Can you work these out from the model? Positions are in its coordinate system, mm. A direction names the side the tool comes from. Round coordinates to 2 decimals unless told otherwise and drop trailing zeros. Write each loop counter-clockwise with the first axis right and the second up, starting at its lowest first coordinate (ties: lowest second). Pieces come first, ordered by that corner, then holes. Notation, with made-up numbers: (48, 56.5) - (89, 56.5) arc R37 ccw to (89, 92.5) - close; hole circle Ø4 at (-29.75, 72.25). An arc over 180 degrees is marked (long way). One line per item, written item: value. Start each with the question number.
(1) On a 3-axis mill with a long thin cutter (end or side, diameter ignored), from which of +Z, -Z, +X, -X, +Y, -Y can I reach the whole of each face in a straight line? I mean faces 1 (the face through (-33, 0, 77.986)), 2 (the face through (-16.92, -0.07, 51.26)). Say none if no direction works.
(2) I want a section at D-D on z = 35. List the corners of the cut face in (x, y) for me.
(3) If I drill on L1, parallel to X at y = -2.5, z = 9; L2, parallel to X at y = -1, z = 51, over which ranges is the centre line in solid material (lowest first)? Write a range as from..to.
(4) I'm going to push a flat-ended pin straight in: pin 1 Ø2 at (y, z) = (-3.5, 18.5) entering from +X. Where does the tip first touch, or does it pass through?
(5) I want a section at C-C on x = -19. Give the number of separate pieces and of enclosed holes in the cut face, plus the area to 3 significant figures.
(6) Thinking about a two-plate mould opening in Z: for faces 3 (the face through (-30, -5.08, 3)), 4 (the face through (-16.9, -0.1, 20.8)), 5 (the face through (-16.92, -0.07, -24.94)), 6 (the face through (-16.81, -0.07, 74.12)), which applies, +Z half, -Z half, draft (parallel to the pull), parting line (faces both ways), or undercut?
(7) I want a section at B-B on z = 5.5. List the corners of the cut face in (x, y) for me, plus the area to 3 significant figures.
(8) I want a section at A-A on y = 0.25. List the corners of the cut face in (x, z) for me, plus the area to 3 significant figures.
from build123d import *

# Parameters (mm, degrees)
F1_DEPTH = 5.08


with BuildPart() as f1:
    # F0 (on Front) → F1 (new body, symmetric)
    with BuildSketch(Plane.XZ):
        Polygon((-20.673906, 77.98629), (-46.073906, 77.98629), (-46.073906, -74.41371), (-20.673906, -74.41371), (-13.053906, -66.79371), (-20.673906, -59.17371), (-13.053906, -51.55371), (-20.673906, -43.93371), (-13.053906, -36.31371), (-20.673906, -28.69371), (-13.053906, -21.07371), (-20.673906, -13.45371), (-13.053906, -5.83371), (-20.673906, 1.78629), (-13.053906, 9.40629), (-20.673906, 17.02629), (-13.053906, 24.64629), (-20.673906, 32.26629), (-13.053906, 39.88629), (-20.673906, 47.50629), (-13.053906, 55.12629), (-20.673906, 62.74629), (-13.053906, 70.36629), align=None)
    extrude(amount=F1_DEPTH, both=True)


solid = f1.part
Established:
1. face 1: +Z, +X, -X, +Y, -Y
1. face 2: +X, +Y, -Y
2. outline: (-46.07, -5.08) - (-17.94, -5.08) - (-17.94, 5.08) - (-46.07, 5.08) - close
3. L1: -46.07..-13.46
3. L2: -46.07..-17.18
4. pin 1: x = -18.2
5. separate pieces: 10
5. enclosed holes: 0
5. area: 1,210 mm2
6. face 3: draft
6. face 4: undercut
6. face 5: undercut
6. face 6: +Z half
7. outline: (-46.07, -5.08) - (-16.96, -5.08) - (-16.96, 5.08) - (-46.07, 5.08) - close
7. area: 296 mm2
8. outline: (-46.07, -74.41) - (-20.67, -74.41) - (-13.05, -66.79) - (-20.67, -59.17) - (-13.05, -51.55) - (-20.67, -43.93) - (-13.05, -36.31) - (-20.67, -28.69) - (-13.05, -21.07) - (-20.67, -13.45) - (-13.05, -5.83) - (-20.67, 1.79) - (-13.05, 9.41) - (-20.67, 17.03) - (-13.05, 24.65) - (-20.67, 32.27) - (-13.05, 39.89) - (-20.67, 47.51) - (-13.05, 55.13) - (-20.67, 62.75) - (-13.05, 70.37) - (-20.67, 77.99) - (-46.07, 77.99) - close
8. area: 4,450 mm2
